Geometry: final body of the model. Coordinates: model frame, mm. A direction names the side the tool comes from. Give positions to 0.01 mm unless a question says otherwise; leave off trailing zeros. Write each loop counter-clockwise with the first axis right and the second up, starting at its lowest first coordinate (ties: lowest second). Pieces come first, ordered by that corner, then holes. Notation, with made-up numbers: (61, 18.25) - (108, 18.25) arc R16 ccw to (108, 23.25) - close; hole circle Ø2 at (-15.75, 52.25). An arc over 180 degrees is marked (long way). Return JSON: item names as keys, results as strings.
from build123d import *

# Parameters (mm, degrees)
SKETCH1_R           = 2.019299997
SKETCH1_R_2         = 2.019299996
SKETCH1_R_3         = 2.070099997
BOSS_EXTRUDE1_DEPTH = 2.54
FILLET2_R           = 2.54


with BuildPart() as part:
    # Sketch1 → Boss-Extrude1 (new body)
    with BuildSketch(Plane.XY):
        Polygon((-12.959899663, -36.98438298), (28.449865782, -44.000886797), (31.100646676, -28.356597569), (56.143695302, -32.599911782), (45.085639298, -97.861973534), (-21.367174772, -86.602155504), align=None)
        with Locations((-6.163136056, -46.554336191)):
            Circle(SKETCH1_R, mode=Mode.SUBTRACT)
        with Locations((-11.467278822, -77.858146974)):
            Circle(SKETCH1_R_2, mode=Mode.SUBTRACT)
        with Locations((18.87991257, -50.797650404)):
            Circle(SKETCH1_R_2, mode=Mode.SUBTRACT)
        with Locations((13.575769804, -82.101461187)):
            Circle(SKETCH1_R_2, mode=Mode.SUBTRACT)
        with Locations((38.318029948, -61.782055276)):
            Circle(SKETCH1_R_3, mode=Mode.SUBTRACT)
        with Locations((34.074715735, -86.825103902)):
            Circle(SKETCH1_R_3, mode=Mode.SUBTRACT)
        with Locations((42.561344161, -36.73900665)):
            Circle(SKETCH1_R_3, mode=Mode.SUBTRACT)
    extrude(amount=BOSS_EXTRUDE1_DEPTH)

    # Fillet2
    fillet2_edges = [part.edges().sort_by_distance(p)[0] for p in [
        (-21.367174772, -86.602155504, 1.27),
        (-12.959899663, -36.98438298, 1.27),
        (28.449865782, -44.000886797, 1.27),
        (31.100646676, -28.356597569, 1.27),
        (56.143695302, -32.599911782, 1.27),
        (45.085639298, -97.861973534, 1.27),
    ]]
    fillet(fillet2_edges, radius=FILLET2_R)


solid = part.part
Q1. Section query B-B, the plane z = 2. Return the cut outline in (x, y).
Answer key:
{"outline": "(-20.94, -84.1) arc R2.54 ccw to (-18.86, -87.03) - (42.58, -97.44) arc R2.54 ccw to (45.51, -95.36) - (55.72, -35.1) arc R2.54 ccw to (53.64, -32.18) - (33.6, -28.78) arc R2.54 ccw to (30.68, -30.86) - (28.87, -41.5) arc R2.54 cw to (25.95, -43.58) - (-10.46, -37.41) arc R2.54 ccw to (-13.38, -39.49) - close; hole circle Ø4.04 at (-11.47, -77.86); hole circle Ø4.04 at (-6.16, -46.55); hole circle Ø4.04 at (13.58, -82.1); hole circle Ø4.04 at (18.88, -50.8); hole circle Ø4.14 at (34.07, -86.83); hole circle Ø4.14 at (38.32, -61.78); hole circle Ø4.14 at (42.56, -36.74)"}
Q2. Material intervals for probe 1 along X at (y, z) = (-49, 0.65); probe 2 along X at (y, z) = (-51.5, 2.1); probe 3 along Y at (x, z) = (12.5, 1.8), sorted ascending. Write a range as [from, to].
Answer key:
{"probe 1": "x = [-15, 17.96], [19.8, 53.36]", "probe 2": "x = [-15.42, 16.99], [20.77, 52.94]", "probe 3": "y = [-92.34, -83.81], [-80.39, -41.3]"}
Q3. Section query D-D, the plane y = -67.5. Return the cut outline in (x, z).
Answer key:
{"outline": "(-18.13, 0) - (50.23, 0) - (50.23, 2.54) - (-18.13, 2.54) - close"}
Q4. Section query A-A, the plane x = 43.5. Return the cut outline in (y, z), plus the area to 3 significant figures.
Answer key:
{"outline": "(-97.42, 0) - (-38.58, 0) - (-38.58, 2.54) - (-97.42, 2.54) - close; (-34.89, 0) - (-30.46, 0) - (-30.46, 2.54) - (-34.89, 2.54) - close", "area": "161 mm^2"}
Q5. Pin query (flat end, axial travel): P1, Ø3.5, axis at x = 42.56, y = -36.74, coming from the -Z side; P2, Ø4.5, axis at x = -6.16, y = -46.55, coming from the -Z side; P3, Ø1.5, axis at x = 37, z = 1, coming from the +Y side; P4, Ø1.5, axis at y = -51.5, z = 0.5, coming from the -X side. Return the tip coordinate at first contact, or that it passes through.
Answer key:
{"P1": "passes through", "P2": "stops at z = 0", "P3": "stops at y = -29.23", "P4": "stops at x = -15.55"}
Q6. Section query C-C, the plane y = -86. Return the cut outline in (x, z).
Answer key:
{"outline": "(-20.5, 0) - (32.18, 0) - (32.18, 2.54) - (-20.5, 2.54) - close; (35.97, 0) - (47.1, 0) - (47.1, 2.54) - (35.97, 2.54) - close"}
Q7. Set-up query: faces 1 (the cylindrical face through (-6.426, -44.552, 1.252)), 2 (the flat face through (7.49, -40.45, 1.25)). Return all of +Z, -Z, +X, -X, +Y, -Y with unobstructed straight access to the full face (end or side cutting, diameter ignored); none if empty.
Answer key:
{"face 1": "+Z, -Z", "face 2": "+Z, -Z, +Y"}
Q8. Mould query, pull axis X, two halves, no side actions, for faces 3 (the flat face through (18, -63, 0)), 4 (the cylindrical face through (13.138, -84.073, 1.252)), 5 (the cylindrical face through (-20.525, -85.97, 1.288)). Classes: pulls with the +X half, pulls with the -X half, needs draft (parallel to the pull), parting line crosses it, or undercut.
Answer key:
{"face 3": "needs draft", "face 4": "undercut", "face 5": "pulls with the -X half"}
